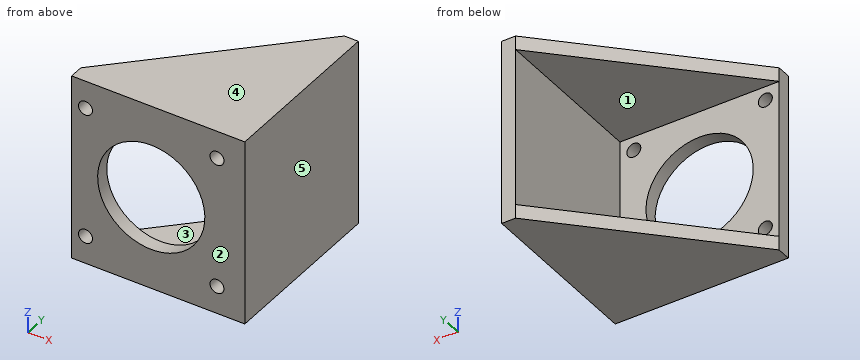
```python
from build123d import *

# Parameters (mm, degrees)
SKETCH1_W           = 57
SKETCH1_H           = 57
SKETCH1_R           = 2.5
SKETCH1_R_2         = 19.2
BOSS_EXTRUDE1_DEPTH = 5
SKETCH2_W           = 5
SKETCH2_H           = 62
BOSS_EXTRUDE2_DEPTH = 57
BOSS_EXTRUDE3_DEPTH = 5
BOSS_EXTRUDE4_START = -57
BOSS_EXTRUDE4_DEPTH = 5


with BuildPart() as part:
    # Sketch1 → Boss-Extrude1 (new body)
    with BuildSketch(Plane(origin=(0, 0, 0), x_dir=(1, 0, 0), z_dir=(0, 1, 0))):
        Rectangle(SKETCH1_W, SKETCH1_H)
        with Locations(Location((-23.55, 23.55, 0), (0, 0, 270))):
            Circle(SKETCH1_R, mode=Mode.SUBTRACT)
        with Locations(Location((23.55, 23.55, 0), (0, 0, 270))):
            Circle(SKETCH1_R, mode=Mode.SUBTRACT)
        with Locations(Location((23.55, -23.55, 0), (0, 0, 270))):
            Circle(SKETCH1_R, mode=Mode.SUBTRACT)
        with Locations(Location((-23.55, -23.55, 0), (0, 0, 270))):
            Circle(SKETCH1_R, mode=Mode.SUBTRACT)
        with Locations(Location((0, 0, 0), (0, 0, 270))):
            Circle(SKETCH1_R_2, mode=Mode.SUBTRACT)
    extrude(amount=BOSS_EXTRUDE1_DEPTH)

    # Sketch2 → Boss-Extrude2 (add)
    with BuildSketch(Plane.XY.offset(28.5)):
        with Locations((31, 31)):
            Rectangle(SKETCH2_W, SKETCH2_H)
    extrude(amount=-BOSS_EXTRUDE2_DEPTH)

    # Sketch3 → Boss-Extrude3 (add)
    with BuildSketch(Plane.XY.offset(28.5)):
        Polygon((28.5, 62), (-28.5, 5), (-28.5, 0), (33.5, 0), (33.5, 62), align=None)
    extrude(amount=BOSS_EXTRUDE3_DEPTH)

    # Sketch3<2> → Boss-Extrude4 (add)
    with BuildSketch(Plane.XY.offset(28.5).offset(BOSS_EXTRUDE4_START)):
        Polygon((28.5, 62), (-28.5, 5), (-28.5, 0), (33.5, 0), (33.5, 62), align=None)
    extrude(amount=-BOSS_EXTRUDE4_DEPTH)


solid = part.part
```
Source: CAD feature listing. Evaluate the final solid. Frame: model axes, mm. Face numbers are marked on the shaded views. A direction names the side the tool comes from. Give positions to 0.01 mm unless a question says otherwise; leave off trailing zeros. Loops run counter-clockwise (first coordinate to the right, second up) from the corner with the lowest first, then second, coordinate; pieces in that order, holes last. Notation, with made-up numbers: (89.5, -1) -> (138.5, -1) arc R18 ccw to (138.5, 7) -> close; hole circle Ø11 at (11.5, -8.5). An arc over 180 degrees is marked (long way). Put each result on its own line as item: value. Start each with the question number.
1) Draft query along Z for the marked faces 3, 4 and 5. Return one class per face: released by +Z, released by -Z, zero draft, split by the parting line, or undercut.
2) Cut plane D-D (z = 23.55). Return loops of the section in (x, y).
3) Cut plane C-C (x = 23.55). Return loops of the section in (y, z).
4) Contact query for flat-ended pins moving along their axis: P1, Ø17, axis at y = 46, z = -7, coming from the -X side; P2, Ø8, axis at x = 23.55, z = -23.55, coming from the -Y side. Output: stop coordinate, or through.
5) Reachability of the marked faces 1 and 2 from +Z, -Z, +X, -X, +Y, -Y: full face, straight path, thin tool, end or side. Return the list, or none.
6) Material intervals for probe 1 along X at (y, z) = (3.5, -23.5); probe 2 along Z at (x, y) = (-23, 2); probe 3 along Z at (x, y) = (15, 26), sorted ascending.
7) Cut plane A-A (x = 0). Return loops of the section in (y, z).
8) Cut plane B-B (z = 0). Return loops of the section in (x, y), then the cut area to 3 significant figures.
Results are:
1. face 3: undercut
1. face 4: released by +Z
1. face 5: zero draft
2. outline: (-28.5, 0) -> (-26.05, 0) -> (-26.05, 5) -> (-28.5, 5) -> close; (-21.05, 0) -> (21.05, 0) -> (21.05, 5) -> (-21.05, 5) -> close; (26.05, 0) -> (33.5, 0) -> (33.5, 62) -> (28.5, 62) -> (28.5, 5) -> (26.05, 5) -> close
3. outline: (0, -33.5) -> (57.05, -33.5) -> (57.05, -28.5) -> (5, -28.5) -> (5, -26.05) -> (0, -26.05) -> close; (0, -21.05) -> (5, -21.05) -> (5, 21.05) -> (0, 21.05) -> close; (0, 26.05) -> (5, 26.05) -> (5, 28.5) -> (57.05, 28.5) -> (57.05, 33.5) -> (0, 33.5) -> close
4. P1: stops at x = 28.5
4. P2: stops at y = 0
5. face 1: -X, +Y
5. face 2: +Z, -Z, +X, -X, -Y
6. probe 1: x = -28.5 to -26.05, -21.05 to 21.05, 26.05 to 33.5
6. probe 2: z = -33.5 to -25.99, -21.11 to 21.11, 25.99 to 33.5
6. probe 3: z = -33.5 to -28.5, 28.5 to 33.5
7. outline: (0, -33.5) -> (33.5, -33.5) -> (33.5, -28.5) -> (5, -28.5) -> (5, -19.2) -> (0, -19.2) -> close; (0, 19.2) -> (5, 19.2) -> (5, 28.5) -> (33.5, 28.5) -> (33.5, 33.5) -> (0, 33.5) -> close
8. outline: (-28.5, 0) -> (-19.2, 0) -> (-19.2, 5) -> (-28.5, 5) -> close; (19.2, 0) -> (33.5, 0) -> (33.5, 62) -> (28.5, 62) -> (28.5, 5) -> (19.2, 5) -> close
8. area: 403 mm2
